Part model, mm, in its own coordinate system. Face numbers are marked on the shaded views. A direction names the side the tool comes from. Give positions to 0.01 mm unless a question says otherwise; leave off trailing zeros. Write each loop counter-clockwise with the first axis right and the second up, starting at its lowest first coordinate (ties: lowest second). Pieces come first, ordered by that corner, then holes. Notation, with made-up numbers: M 46.5,-10 L 56.5,-10 A17 ccw 56.5,17 Z; hole C -17,79.25 d7. An arc over 180 degrees is marked long. Answer as CSV lines item,"result". Start each with the question number.
Item 1: Band-saw the part on D-D, the plane x = 31. List the corners of the cut face in (y, z).
Item 2: Pin check, flat tips, straight feed: pin 1 (6 mm diameter, centred on x = 25.5, z = 5.5, fed in from -Y); pin 2 (1 mm diameter, centred on y = -9.5, z = 7.5, fed in from +X); pin 3 (3 mm diameter, centred on y = -32, z = 3, fed in from +X). Stop position of each tip, or through.
Item 3: Two-plate mould, pull along Y, no slides. Class the marked faces 1, 2, 3 and 4: +Y half, -Y half, draft (parallel to the pull), parting line (faces both ways), or undercut.
Item 4: Band-saw the part on C-C, the plane x = -37. List the corners of the cut face in (y, z).
Item 5: Band-saw the part on B-B, the plane y = -31. List the corners of the cut face in (x, z), then the cut area to 3 significant figures.
Item 6: 3-axis set-ups, long thin cutter, end or side, ignore diameter. For the marked faces 5 and 6: which of +Z, -Z, +X, -X, +Y, -Y reach the whole face in a straight line?
Item 7: Band-saw the part on A-A, the plane z = 5.25. List the corners of the cut face in (x, y).
Item 8: Wall check: L1, parallel to Y at x = -40, z = 6.5; L2, parallel to Y at x = -42.5, z = 5.5; L3, parallel to X at y = 9.5, z = 1.5. Give the ranges that are in metal, low to high. Write a range as from..to.
from build123d import *

# Parameters (mm, degrees)
F0_R     = 4.5
F1_DEPTH = 12


with BuildPart() as f1:
    # F0 (on Top) → F1 (new body)
    with BuildSketch(Plane.XY):
        with BuildLine():
            ThreePointArc((0, -10), (2.928932, -2.928932), (10, 0))
            Line((10, 0), (35, 0))
            ThreePointArc((35, 0), (42.071068, 2.928932), (45, 10))
            Line((45, 10), (45, 20))
            ThreePointArc((45, 20), (42.071068, 27.071068), (35, 30))
            Line((35, 30), (-40, 30))
            ThreePointArc((-40, 30), (-47.071068, 27.071068), (-50, 20))
            Line((-50, 20), (-50, -30))
            ThreePointArc((-50, -30), (-47.071068, -37.071068), (-40, -40))
            Line((-40, -40), (-10, -40))
            ThreePointArc((-10, -40), (-2.928932, -37.071068), (0, -30))
            Line((0, -30), (0, -10))
        make_face()
        with Locations((-40, -30)):
            Circle(F0_R, mode=Mode.SUBTRACT)
        with Locations((-40, 20)):
            Circle(F0_R, mode=Mode.SUBTRACT)
    extrude(amount=F1_DEPTH)


solid = f1.part
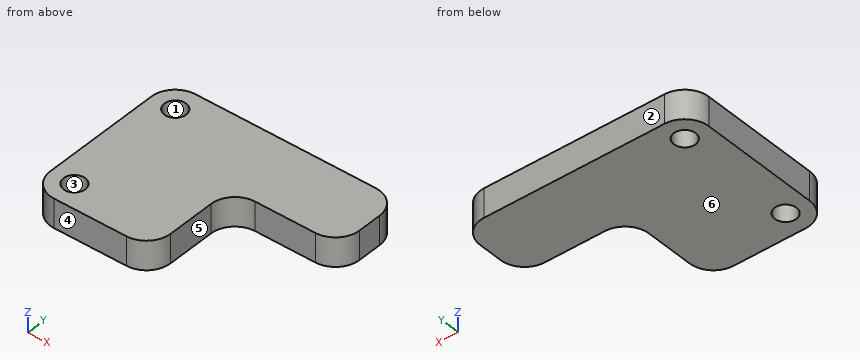
Output:
1,outline,"M 0,0 L 30,0 L 30,12 L 0,12 Z"
2,pin 1,"y = 0"
2,pin 2,"x = 0.05"
2,pin 3,"x = -0.01"
3,face 1,"undercut"
3,face 2,"+Y half"
3,face 3,"undercut"
3,face 4,"-Y half"
4,outline,"M -40,0 L -33.35,0 L -33.35,12 L -40,12 Z; M -26.65,0 L 16.65,0 L 16.65,12 L -26.65,12 Z; M 23.35,0 L 30,0 L 30,12 L 23.35,12 Z"
5,outline,"M -49.95,0 L -44.39,0 L -44.39,12 L -49.95,12 Z; M -35.61,0 L -0.05,0 L -0.05,12 L -35.61,12 Z"
5,area,"493 mm²"
6,face 5,"+Z, -Z, +X, -Y"
6,face 6,"-Z, +X, -X, +Y, -Y"
7,outline,"M -50,-30 A10 ccw -40,-40 L -10,-40 A10 ccw 0,-30 L 0,-10 A10 cw 10,0 L 35,0 A10 ccw 45,10 L 45,20 A10 ccw 35,30 L -40,30 A10 ccw -50,20 Z; hole C -40,-30 d9; hole C -40,20 d9"
8,L1,"-40..-34.5, -25.5..15.5, 24.5..30"
8,L2,"-39.68..-33.74, -26.26..16.26, 23.74..29.68"
8,L3,"-50..44.99"
